```python
from build123d import *

# Parameters (mm, degrees)
IZIM1_R                     = 12.5
Y_KSEKLIK_EKSTR_ZYON1_DEPTH = 30
IZIM2_R                     = 5
KES_EKSTR_ZYON1_DEPTH       = 25
PAH1_SIZE                   = 0.5


with BuildPart() as part:
    # Çizim1 → Yükseklik-Ekstrüzyon1 (new body)
    with BuildSketch(Plane.XY):
        Circle(IZIM1_R)
    extrude(amount=Y_KSEKLIK_EKSTR_ZYON1_DEPTH)

    # Çizim2 → Kes-Ekstrüzyon1 (cut)
    with BuildSketch(Plane.XY.offset(30)):
        Circle(IZIM2_R)
    extrude(amount=-KES_EKSTR_ZYON1_DEPTH, mode=Mode.SUBTRACT)

    # Pah1
    pah1_edges = [part.edges().sort_by_distance(p)[0] for p in [
        (-12.5, 0, 0),
        (-12.5, 0, 30),
        (-5, 0, 30),
    ]]
    chamfer(pah1_edges, length=PAH1_SIZE)


solid = part.part
```
Geometry check sheet. Reference: the model listing, model coordinates, mm. A direction names the side the tool comes from. Coordinates: 2 decimals unless noted, no trailing zeros. Order: outer loops, then holes, each group sorted by start corner. A loop starts at its lowest first (then second) coordinate and runs counter-clockwise, first axis right, second up. Notation, with made-up numbers: (-10, 61) - (17, 61) arc R24 ccw to (17, 80) - close; hole circle Ø9 at (-20, 2.25). An arc over 180 degrees is marked (long way). Use one line per item in the form item = value.
1. Section check A-A (y = 0). Record the boundary of the cut face in (x, z).
Here are the results:
outline = (-12.5, 0.5) - (-12, 0) - (12, 0) - (12.5, 0.5) - (12.5, 29.5) - (12, 30) - (5.5, 30) - (5, 29.5) - (5, 5) - (-5, 5) - (-5, 29.5) - (-5.5, 30) - (-12, 30) - (-12.5, 29.5) - close
2. Gauge pin test, flat ends, axial feed: pin 1 (1 mm diameter, centred on x = 0, y = 1.5, fed in from +Z); pin 2 (1.5 mm diameter, centred on y = 6, z = 15.5, fed in from -X); pin 3 (12 mm diameter, centred on y = -7.5, z = 19, fed in from +X). Record the tip position at first contact, or that the pin passes through.
Here are the results:
pin_1 = 5
pin_2 = -11.34
pin_3 = 12.41
3. Access from +Z, -Z, +X, -X, +Y, -Y to the whole of each face (thin tool, end or side, straight path). Record for faces 1 (the face through (0, 0, 0)), 2 (the face through (-1.08, -4.88, 17.42)).
Here are the results:
face_1 = -Z, +X, -X, +Y, -Y
face_2 = +Z
4. Section check D-D (z = 2). Record the boundary of the cut face in (x, y), then the cut area to 3 significant figures.
Here are the results:
outline = circle Ø25 at (0, 0)
area = 491 mm²
5. Section check C-C (z = 20). Record the boundary of the cut face in (x, y).
Here are the results:
outline = circle Ø25 at (0, 0); hole circle Ø10 at (0, 0)
6. Scan lines: line 1 (Y direction, x = 0, z = 24); line 2 (X direction, y = 0.25, z = 11.5); line 3 (Y direction, x = 3, z = 24). Record each from-to range of solid material in increasing order.
Here are the results:
line_1 = -12.5 to -5, 5 to 12.5
line_2 = -12.5 to -4.99, 4.99 to 12.5
line_3 = -12.13 to -4, 4 to 12.13
